Verification items for this drawing (mm, ordinates from the low corner). A direction names the side the tool comes from. Give positions to 0.01 mm unless a question says otherwise; leave off trailing zeros. Order: outer loops, then holes, each group sorted by start corner. A loop starts at its lowest first (then second) coordinate and runs counter-clockwise, first axis right, second up. Notation, with made-up numbers: (6.5, 55.25) - (26.5, 55.25) arc R22 cw to (26.5, 92.25) - close; hole circle Ø8 at (-12, 88.5). An arc over 180 degrees is marked (long way). Put each result on its own line as item: value. Start each with the question number.
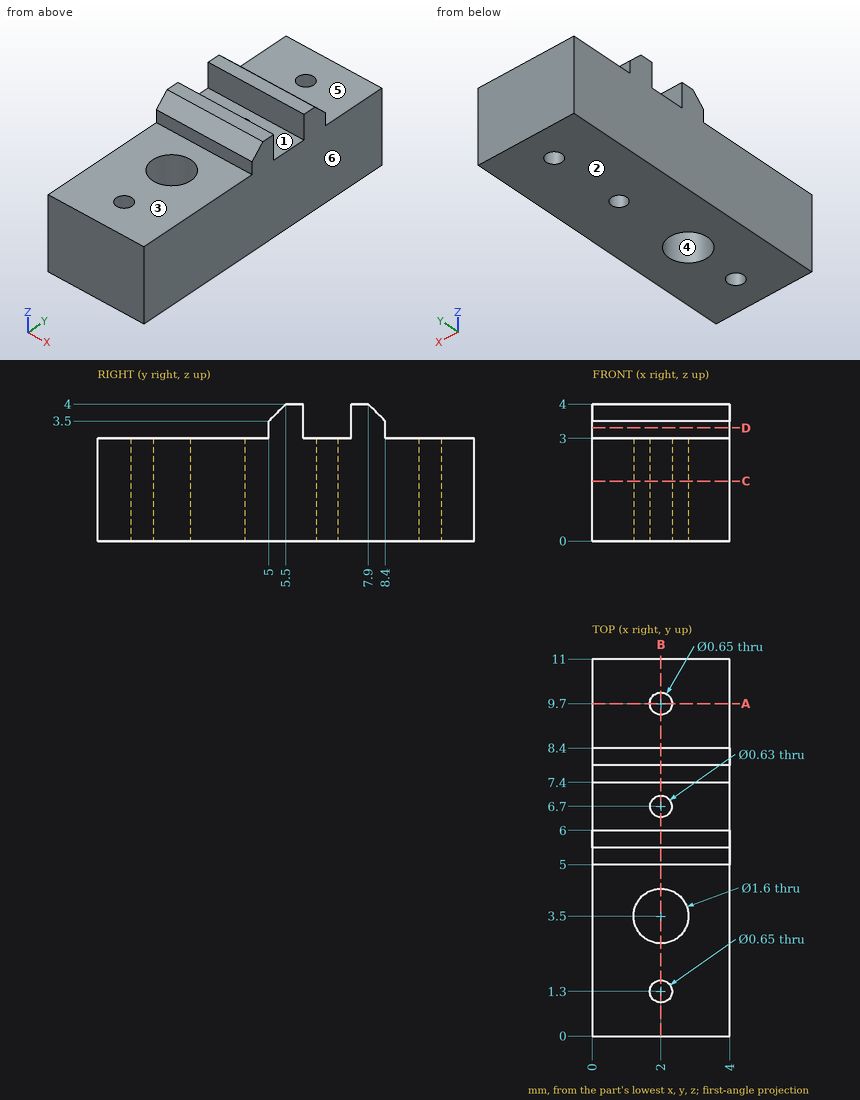
Item 1: Set-up check for the marked faces 1, 2 and 3: record each of +Z, -Z, +X, -X, +Y, -Y from which the full face is reachable in a straight line by a thin tool's end or side.
Item 2: Cross-section at A-A (y = 9.7). Enter the section's corners in (x, z) (3 decimals).
Item 3: Cross-section at C-C (z = 1.75). Enter the section's corners in (x, y) (3 decimals), and give its area (3 significant figures).
Item 4: Thickness scan on line 1 along Y through (x, z) = (2, 1.35) (3 decimals); line 2 along X through (y, z) = (3.5, 1.05); line 3 along Y through (x, z) = (2.2, 1.1). Record the ranges inside material, lowest first.
Item 5: Release check for a two-part mould opening along X. For the marked faces 4, 5 and 6 record: +X half, -X half, draft (parallel to the pull), parting line (faces both ways), or undercut.
Item 6: Gauge pin test, flat end, axial feed: pin 1 Ø0.7 at (x, y) = (2.5, 6.5) entering from +Z. Record the tip position at first contact, or that the pin passes through.
Item 7: Cross-section at D-D (z = 3.3). Enter the section's corners in (x, y), and give its area (3 significant figures).
Item 8: Cross-section at B-B (x = 2). Count the separate pieces of the cut face and the enclosed holes in it, and give its area (3 significant figures).
Recorded:
1. face 1: +Z, +X, -X
1. face 2: -Z, +X, -X, +Y, -Y
1. face 3: +Z, +X, -X, -Y
2. outline: (0, 0) - (1.675, 0) - (1.675, 3) - (0, 3) - close; (2.325, 0) - (4, 0) - (4, 3) - (2.325, 3) - close
3. outline: (0, 0) - (4, 0) - (4, 11) - (0, 11) - close; hole circle Ø1.6 at (2, 3.5); hole circle Ø0.65 at (2, 1.3); hole circle Ø0.65 at (2, 9.7); hole circle Ø0.63 at (2, 6.7)
3. area: 41.0 mm^2
4. line 1: y = 0 to 0.975, 1.625 to 2.7, 4.3 to 6.385, 7.015 to 9.375, 10.025 to 11
4. line 2: x = 0 to 1.2, 2.8 to 4
4. line 3: y = 0 to 1.04, 1.56 to 2.73, 4.27 to 6.46, 6.94 to 9.44, 9.96 to 11
5. face 4: undercut
5. face 5: draft
5. face 6: +X half
6. pin 1: stops at z = 3
7. outline: (0, 5) - (4, 5) - (4, 6) - (0, 6) - close; (0, 7.4) - (4, 7.4) - (4, 8.4) - (0, 8.4) - close
7. area: 8.00 mm^2
8. separate pieces: 5
8. enclosed holes: 0
8. area: 24.2 mm^2
